```python
from build123d import *

# Parameters (mm, degrees)
SKETCH_1_W      = 29
SKETCH_1_H      = 12.7
EXTRUDE_1_DEPTH = 15.7
EXTRUDE_2_DEPTH = 3.5
FILLET_1_R      = 0.05
CHAMFER_1_SIZE  = 1.5
FILLET_2_R      = 0.75


with BuildPart() as part:
    # Эскиз1 → Бобышка-Вытянуть1 (new body)
    with BuildSketch(Plane(origin=(0, 0, 0), x_dir=(1, 0, 0), z_dir=(0, 1, 0))):
        Rectangle(SKETCH_1_W, SKETCH_1_H)
    extrude(amount=EXTRUDE_1_DEPTH)

    # Эскиз2 → Бобышка-Вытянуть2 (add)
    with BuildSketch(Plane.XZ):
        with BuildLine():
            Line((-12.3, 4.15), (-11.9, 4.15))
            ThreePointArc((-11.9, 4.15), (-11.864644661, 4.135355339), (-11.85, 4.1))
            Line((-11.85, 4.1), (-11.85, 3.4))
            ThreePointArc((-11.85, 3.4), (-11.864644661, 3.364644661), (-11.9, 3.35))
            Line((-11.9, 3.35), (-12.3, 3.35))
            ThreePointArc((-12.3, 3.35), (-12.335355339, 3.364644661), (-12.35, 3.4))
            Line((-12.35, 3.4), (-12.35, 4.1))
            ThreePointArc((-12.35, 4.1), (-12.335355339, 4.135355339), (-12.3, 4.15))
        make_face()
        with BuildLine():
            Line((2.65, 4.1), (2.65, 3.4))
            ThreePointArc((2.65, 3.4), (2.664644661, 3.364644661), (2.7, 3.35))
            Line((2.7, 3.35), (3.1, 3.35))
            ThreePointArc((3.1, 3.35), (3.135355339, 3.364644661), (3.15, 3.4))
            Line((3.15, 3.4), (3.15, 4.1))
            ThreePointArc((3.15, 4.1), (3.135355339, 4.135355339), (3.1, 4.15))
            Line((3.1, 4.15), (2.7, 4.15))
            ThreePointArc((2.7, 4.15), (2.664644661, 4.135355339), (2.65, 4.1))
        make_face()
        with BuildLine():
            Line((7.65, 4.1), (7.65, 3.4))
            ThreePointArc((7.65, 3.4), (7.664644661, 3.364644661), (7.7, 3.35))
            Line((7.7, 3.35), (8.1, 3.35))
            ThreePointArc((8.1, 3.35), (8.135355339, 3.364644661), (8.15, 3.4))
            Line((8.15, 3.4), (8.15, 4.1))
            ThreePointArc((8.15, 4.1), (8.135355339, 4.135355339), (8.1, 4.15))
            Line((8.1, 4.15), (7.7, 4.15))
            ThreePointArc((7.7, 4.15), (7.664644661, 4.135355339), (7.65, 4.1))
        make_face()
        with BuildLine():
            Line((12.65, 4.1), (12.65, 3.4))
            ThreePointArc((12.65, 3.4), (12.664644661, 3.364644661), (12.7, 3.35))
            Line((12.7, 3.35), (13.1, 3.35))
            ThreePointArc((13.1, 3.35), (13.135355339, 3.364644661), (13.15, 3.4))
            Line((13.15, 3.4), (13.15, 4.1))
            ThreePointArc((13.15, 4.1), (13.135355339, 4.135355339), (13.1, 4.15))
            Line((13.1, 4.15), (12.7, 4.15))
            ThreePointArc((12.7, 4.15), (12.664644661, 4.135355339), (12.65, 4.1))
        make_face()
        with BuildLine():
            Line((2.65, -3.4), (2.65, -4.1))
            ThreePointArc((2.65, -4.1), (2.664644661, -4.135355339), (2.7, -4.15))
            Line((2.7, -4.15), (3.1, -4.15))
            ThreePointArc((3.1, -4.15), (3.135355339, -4.135355339), (3.15, -4.1))
            Line((3.15, -4.1), (3.15, -3.4))
            ThreePointArc((3.15, -3.4), (3.135355339, -3.364644661), (3.1, -3.35))
            Line((3.1, -3.35), (2.7, -3.35))
            ThreePointArc((2.7, -3.35), (2.664644661, -3.364644661), (2.65, -3.4))
        make_face()
        with BuildLine():
            Line((7.65, -3.4), (7.65, -4.1))
            ThreePointArc((7.65, -4.1), (7.664644661, -4.135355339), (7.7, -4.15))
            Line((7.7, -4.15), (8.1, -4.15))
            ThreePointArc((8.1, -4.15), (8.135355339, -4.135355339), (8.15, -4.1))
            Line((8.15, -4.1), (8.15, -3.4))
            ThreePointArc((8.15, -3.4), (8.135355339, -3.364644661), (8.1, -3.35))
            Line((8.1, -3.35), (7.7, -3.35))
            ThreePointArc((7.7, -3.35), (7.664644661, -3.364644661), (7.65, -3.4))
        make_face()
        with BuildLine():
            Line((12.65, -3.4), (12.65, -4.1))
            ThreePointArc((12.65, -4.1), (12.664644661, -4.135355339), (12.7, -4.15))
            Line((12.7, -4.15), (13.1, -4.15))
            ThreePointArc((13.1, -4.15), (13.135355339, -4.135355339), (13.15, -4.1))
            Line((13.15, -4.1), (13.15, -3.4))
            ThreePointArc((13.15, -3.4), (13.135355339, -3.364644661), (13.1, -3.35))
            Line((13.1, -3.35), (12.7, -3.35))
            ThreePointArc((12.7, -3.35), (12.664644661, -3.364644661), (12.65, -3.4))
        make_face()
        with BuildLine():
            Line((-12.35, -3.4), (-12.35, -4.1))
            ThreePointArc((-12.35, -4.1), (-12.335355339, -4.135355339), (-12.3, -4.15))
            Line((-12.3, -4.15), (-11.9, -4.15))
            ThreePointArc((-11.9, -4.15), (-11.864644661, -4.135355339), (-11.85, -4.1))
            Line((-11.85, -4.1), (-11.85, -3.4))
            ThreePointArc((-11.85, -3.4), (-11.864644661, -3.364644661), (-11.9, -3.35))
            Line((-11.9, -3.35), (-12.3, -3.35))
            ThreePointArc((-12.3, -3.35), (-12.335355339, -3.364644661), (-12.35, -3.4))
        make_face()
    extrude(amount=EXTRUDE_2_DEPTH)

    # Скругление1
    fillet_1_edges = [part.edges().sort_by_distance(p)[0] for p in [
        (2.664644661, -3.5, -4.135355339),
        (2.9, -3.5, -4.15),
        (3.135355339, -3.5, -4.135355339),
        (3.15, -3.5, -3.75),
        (3.135355339, -3.5, -3.364644661),
        (2.9, -3.5, -3.35),
        (2.664644661, -3.5, -3.364644661),
        (2.65, -3.5, -3.75),
        (7.664644661, -3.5, -4.135355339),
        (7.9, -3.5, -4.15),
        (8.135355339, -3.5, -4.135355339),
        (8.15, -3.5, -3.75),
        (8.135355339, -3.5, -3.364644661),
        (7.9, -3.5, -3.35),
        (7.664644661, -3.5, -3.364644661),
        (7.65, -3.5, -3.75),
        (12.664644661, -3.5, -4.135355339),
        (12.9, -3.5, -4.15),
        (13.135355339, -3.5, -4.135355339),
        (13.15, -3.5, -3.75),
        (13.135355339, -3.5, -3.364644661),
        (12.9, -3.5, -3.35),
        (12.664644661, -3.5, -3.364644661),
        (12.65, -3.5, -3.75),
        (-12.335355339, -3.5, -4.135355339),
        (-12.1, -3.5, -4.15),
        (-11.864644661, -3.5, -4.135355339),
        (-11.85, -3.5, -3.75),
        (-11.864644661, -3.5, -3.364644661),
        (-12.1, -3.5, -3.35),
        (-12.335355339, -3.5, -3.364644661),
        (-12.35, -3.5, -3.75),
        (-12.335355339, -3.5, 3.364644661),
        (-12.1, -3.5, 3.35),
        (-11.864644661, -3.5, 3.364644661),
        (-11.85, -3.5, 3.75),
        (-11.864644661, -3.5, 4.135355339),
        (-12.1, -3.5, 4.15),
        (-12.335355339, -3.5, 4.135355339),
        (-12.35, -3.5, 3.75),
        (2.664644661, -3.5, 3.364644661),
        (2.9, -3.5, 3.35),
        (3.135355339, -3.5, 3.364644661),
        (3.15, -3.5, 3.75),
        (3.135355339, -3.5, 4.135355339),
        (2.9, -3.5, 4.15),
        (2.664644661, -3.5, 4.135355339),
        (2.65, -3.5, 3.75),
        (7.664644661, -3.5, 3.364644661),
        (7.9, -3.5, 3.35),
        (8.135355339, -3.5, 3.364644661),
        (8.15, -3.5, 3.75),
        (8.135355339, -3.5, 4.135355339),
        (7.9, -3.5, 4.15),
        (7.664644661, -3.5, 4.135355339),
        (7.65, -3.5, 3.75),
        (12.664644661, -3.5, 3.364644661),
        (12.9, -3.5, 3.35),
        (13.135355339, -3.5, 3.364644661),
        (13.15, -3.5, 3.75),
        (13.135355339, -3.5, 4.135355339),
        (12.9, -3.5, 4.15),
        (12.664644661, -3.5, 4.135355339),
        (12.65, -3.5, 3.75),
    ]]
    fillet(fillet_1_edges, radius=FILLET_1_R)

    # Фаска1
    chamfer_1_edges = [part.edges().sort_by_distance(p)[0] for p in [
        (14.5, 15.7, 0),
    ]]
    chamfer(chamfer_1_edges, length=CHAMFER_1_SIZE)

    # Скругление2
    fillet_2_edges = [part.edges().sort_by_distance(p)[0] for p in [
        (-14.5, 15.7, 0),
        (-0.75, 15.7, 6.35),
        (-0.75, 15.7, -6.35),
        (13, 15.7, 0),
        (14.5, 7.1, -6.35),
        (13.75, 14.95, -6.35),
        (14.5, 7.1, 6.35),
        (14.5, 14.2, 0),
        (13.75, 14.95, 6.35),
        (-14.5, 7.85, 6.35),
        (-14.5, 7.85, -6.35),
    ]]
    fillet(fillet_2_edges, radius=FILLET_2_R)


solid = part.part
```
Source: CAD feature listing. Evaluate the final solid. Frame: model axes, mm. Round coordinates to 2 decimals unless told otherwise and drop trailing zeros. Loops run counter-clockwise (first coordinate to the right, second up) from the corner with the lowest first, then second, coordinate; pieces in that order, holes last.
(1) Section query C-C (y = -1.5). Give the number of separate pieces and of enclosed holes in the cut face, and give its area (3 significant figures).
From the geometry:
separate pieces: 8
enclosed holes: 0
area: 3.18 mm2
(2) Section query B-B (x = 10). Output: boundary loops of the cut face in (y, z), and give its area (3 significant figures).
From the geometry:
outline: (0, -6.35) - (14.95, -6.35) arc R0.75 ccw to (15.7, -5.6) - (15.7, 5.6) arc R0.75 ccw to (14.95, 6.35) - (0, 6.35) - close
area: 199 mm2
(3) Section query A-A (z = 1). Output: boundary loops of the cut face in (x, y).
From the geometry:
outline: (-14.5, 0) - (14.5, 0) - (14.5, 13.89) arc R0.75 ccw to (14.28, 14.42) - (13.22, 15.48) arc R0.75 ccw to (12.69, 15.7) - (-13.75, 15.7) arc R0.75 ccw to (-14.5, 14.95) - close
(4) Contact query for flat-ended pins moving along their axis: pin 1 Ø0.8 at (y, z) = (-2, 3.5) entering from -X; pin 2 Ø0.6 at (y, z) = (-2, -4) entering from +X. Output: stop coordinate, or through.
From the geometry:
pin 1: stops at x = -12.35
pin 2: stops at x = 13.15
(5) Material intervals for probe 1 along Y at (x, z) = (11.25, -0.5); probe 2 along Y at (x, z) = (13.25, 3); probe 3 along X at (y, z) = (14.25, 3.75), sorted ascending.
From the geometry:
probe 1: y = 0 to 15.7
probe 2: y = 0 to 15.45
probe 3: x = -14.5 to 14.41
